```python
from build123d import *

# Parameters (mm, degrees)
SKETCH1_W           = 15.875
SKETCH1_H           = 20.193
SKETCH1_R           = 1.5875
BOSS_EXTRUDE1_DEPTH = 13.208
SKETCH4_W           = 1.778
SKETCH4_H           = 20.193
CUT_EXTRUDE1_DEPTH  = 9.779


with BuildPart() as part:
    # Sketch1 → Boss-Extrude1 (new body)
    with BuildSketch(Plane(origin=(0, 0, 0), x_dir=(0, 0, -1), z_dir=(1, 0, 0))):
        with Locations((7.9375, 10.0965)):
            Rectangle(SKETCH1_W, SKETCH1_H)
        with Locations(Location((13.335, 17.653, 0), (0, 0, 180))):
            Circle(SKETCH1_R, mode=Mode.SUBTRACT)
    extrude(amount=BOSS_EXTRUDE1_DEPTH)

    # Sketch4 → Cut-Extrude1 (cut)
    with BuildSketch(Plane(origin=(0, 0, -15.875), x_dir=(-1, 0, 0), z_dir=(0, 0, -1))):
        with Locations((-5.969, 10.0965)):
            Rectangle(SKETCH4_W, SKETCH4_H)
    extrude(amount=-CUT_EXTRUDE1_DEPTH, mode=Mode.SUBTRACT)


solid = part.part
```
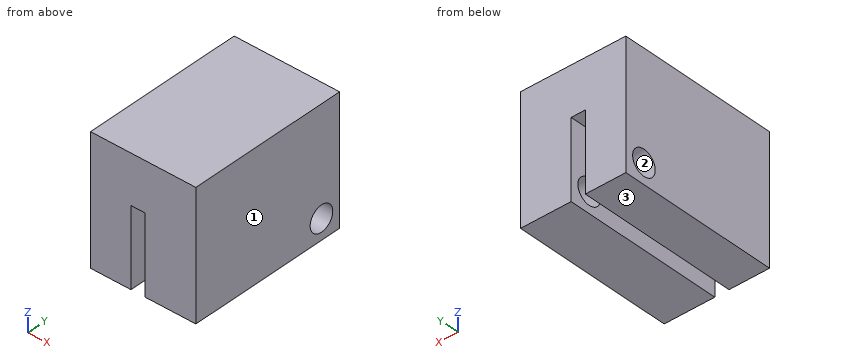
Input: part model. Units: mm. Frame: model coordinates. Face numbers are marked on the shaded views. Round coordinates to 2 decimals unless told otherwise and drop trailing zeros. Write each loop counter-clockwise with the first axis right and the second up, starting at its lowest first coordinate (ties: lowest second). Pieces come first, ordered by that corner, then holes. Notation, with made-up numbers: (84, 30.25) -> (143, 30.25) arc R14 ccw to (143, 54.25) -> close; hole circle Ø1 at (25.25, -29). An arc over 180 degrees is marked (long way). Answer as CSV lines item,"result".
1. Contact query for a flat-ended pin moving along its axis: P1, Ø0.9, axis at x = 6, y = 7.5, coming from the -Z side. Output: stop coordinate, or through.
Geometry says:
P1,"stops at z = -6.1"
2. Section A-A (z = -6.75). Return the cut outline in (x, y).
Geometry says:
outline,"(0, 0) -> (5.08, 0) -> (5.08, 20.19) -> (0, 20.19) -> close; (6.86, 0) -> (13.21, 0) -> (13.21, 20.19) -> (6.86, 20.19) -> close"
3. Ray query, L1, parallel to X at y = 1.5, z = -12.5; L2, parallel to Z at x = 6, y = 1.25; L3, parallel to Y at x = 3.5, z = -12.75. Return the intervals inside material, ascending. Write a range as [from, to].
Geometry says:
L1,"x = [0, 5.08], [6.86, 13.21]"
L2,"z = [-6.1, 0]"
L3,"y = [0, 16.18], [19.13, 20.19]"
4. Section B-B (y = 18.5). Return the cut outline in (x, z) (3 decimals).
Geometry says:
outline,"(0, -15.875) -> (5.08, -15.875) -> (5.08, -14.678) -> (0, -14.678) -> close; (0, -11.992) -> (5.08, -11.992) -> (5.08, -6.096) -> (6.858, -6.096) -> (6.858, -11.992) -> (13.208, -11.992) -> (13.208, 0) -> (0, 0) -> close; (6.858, -15.875) -> (13.208, -15.875) -> (13.208, -14.678) -> (6.858, -14.678) -> close"
5. Section D-D (y = 13.25). Return the cut outline in (x, z) (3 decimals), plus the area to 3 significant figures.
Geometry says:
outline,"(0, -15.875) -> (5.08, -15.875) -> (5.08, -6.096) -> (6.858, -6.096) -> (6.858, -15.875) -> (13.208, -15.875) -> (13.208, 0) -> (0, 0) -> close"
area,"192 mm^2"
6. Section C-C (z = -14.5). Return the cut outline in (x, y), plus the area to 3 significant figures.
Geometry says:
outline,"(0, 0) -> (5.08, 0) -> (5.08, 16.57) -> (0, 16.57) -> close; (0, 18.73) -> (5.08, 18.73) -> (5.08, 20.19) -> (0, 20.19) -> close; (6.86, 0) -> (13.21, 0) -> (13.21, 16.57) -> (6.86, 16.57) -> close; (6.86, 18.73) -> (13.21, 18.73) -> (13.21, 20.19) -> (6.86, 20.19) -> close"
area,"206 mm^2"
7. Mould query, pull axis Z, two halves, no side actions, for the marked faces 1, 2 and 3. Classes: +Z half, -Z half, draft (parallel to the pull), parting line (faces both ways), or undercut.
Geometry says:
face 1,"draft"
face 2,"undercut"
face 3,"-Z half"
